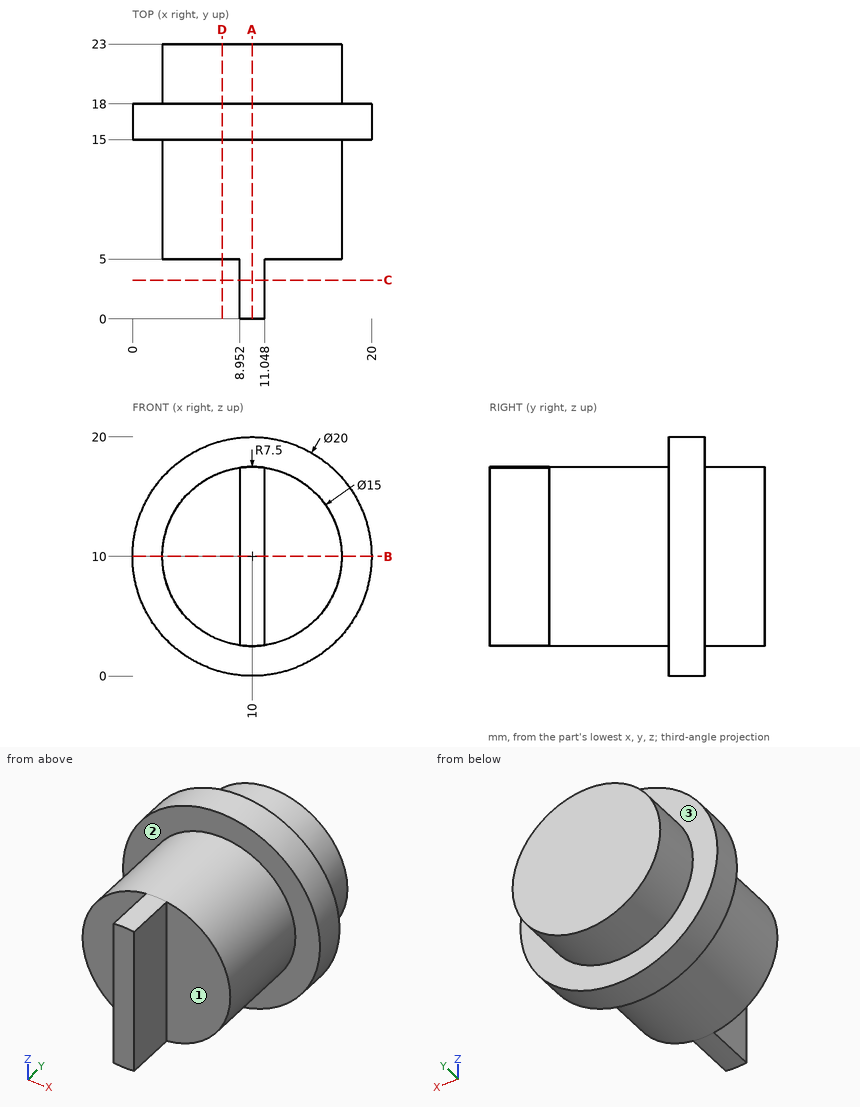
Can you work these out from the drawing? Everything is in mm from the part's minimum corner. A direction names the side the tool comes from. Coordinates: 2 decimals unless noted, no trailing zeros. Loops run counter-clockwise (first coordinate to the right, second up) from the corner with the lowest first, then second, coordinate; pieces in that order, holes last.
1) Imagine slicing it at C-C on y = 3.25. List the corners of the cut face in (x, z) for me.
2) For pin 1 (5 mm diameter, centred on y = 14.5, z = 15, fed in from +X); pin 2 (1 mm diameter, centred on y = 19.5, z = 8.5, fed in from -X); pin 3 (3 mm diameter, centred on x = 5.5, z = 6.5, fed in from -Y), each with a flat end and sliding along its axis, tell me the tip position at first contact or that it passes through.
3) I need wall thicknesses on probe 1 along Y at (x, z) = (4.5, 15.5); probe 2 along X at (y, z) = (12.5, 9.75); probe 3 along X at (y, z) = (2.25, 3). Which ranges of each line are inside material? Lowest first, please.
4) Imagine slicing it at D-D on x = 7.5. List the corners of the cut face in (y, z) for me, plus the area to 3 significant figures.
5) Imagine slicing it at B-B on z = 10. List the corners of the cut face in (x, y) for me, plus the area to 4 significant figures.
6) Which directions (+Z, -Z, +X, -X, +Y, -Y) give clear straight access to the entire face, cutting with the end or side of a thin tool? Please do the marked faces 1, 2 and 3.
7) Imagine slicing it at A-A on x = 10. List the corners of the cut face in (y, z) for me, plus the area to 3 significant figures.
Completed:
1. outline: (8.95, 2.57) arc R7.5 ccw to (11.05, 2.57) - (11.05, 17.43) arc R7.5 ccw to (8.95, 17.43) - close
2. pin 1: stops at x = 19.67
2. pin 2: stops at x = 2.57
2. pin 3: stops at y = 5
3. probe 1: y = 15 to 18
3. probe 2: x = 2.5 to 17.5
3. probe 3: x = 8.95 to 11.05
4. outline: (5, 2.93) - (15, 2.93) - (15, 0.32) - (18, 0.32) - (18, 2.93) - (23, 2.93) - (23, 17.07) - (18, 17.07) - (18, 19.68) - (15, 19.68) - (15, 17.07) - (5, 17.07) - close
4. area: 270 mm2
5. outline: (0, 15) - (2.5, 15) - (2.5, 5) - (8.95, 5) - (8.95, 0) - (11.05, 0) - (11.05, 5) - (17.5, 5) - (17.5, 15) - (20, 15) - (20, 18) - (17.5, 18) - (17.5, 23) - (2.5, 23) - (2.5, 18) - (0, 18) - close
5. area: 295.5 mm2
6. face 1: +Z, -Z, +X, -Y
6. face 2: -Y
6. face 3: +Y
7. outline: (0, 2.5) - (15, 2.5) - (15, 0) - (18, 0) - (18, 2.5) - (23, 2.5) - (23, 17.5) - (18, 17.5) - (18, 20) - (15, 20) - (15, 17.5) - (0, 17.5) - close
7. area: 360 mm2
